Read the model definition and answer for the solid it produces. Units are mm, in the model's axes. Face numbers are marked on the shaded views. A direction names the side the tool comes from. Coordinates: 2 decimals unless noted, no trailing zeros. Loops run counter-clockwise (first coordinate to the right, second up) from the corner with the lowest first, then second, coordinate; pieces in that order, holes last. Notation, with made-up numbers: (-27, 11.5) -> (3, 11.5) arc R38 cw to (3, 49.5) -> close; hole circle Ø3 at (26, 59.5). An arc over 180 degrees is marked (long way). Answer in a Markdown table with one row per item.
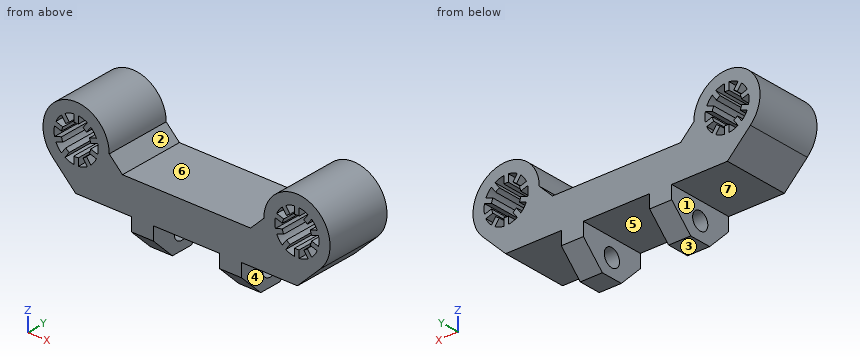
```python
from build123d import *

# Parameters (mm, degrees)
SKETCH1_R                      = 7.5
SKETCH1_R_2                    = 5
SKETCH1_W                      = 5
SKETCH1_H                      = 8
BOSS_EXTRUDE1_DEPTH            = 15
CHAMFER1_SIZE                  = 5
CUT_EXTRUDE1_REACH             = 42.293
SKETCH3_R                      = 2
CUT_EXTRUDE1_DIRECTION_2_REACH = 42.293


with BuildPart() as part:
    # Sketch1 → Boss-Extrude1 (new body)
    # profile 1 of 13: a face of its own
    with BuildSketch(Plane(origin=(0, 0, 0), x_dir=(1, 0, 0), z_dir=(0, 1, 0))):
        with Locations((-25, 0)):
            Circle(SKETCH1_R)
        with Locations((-25, 0)):
            Circle(SKETCH1_R_2, mode=Mode.SUBTRACT)
    # profile 2 of 13: a face of its own
    with BuildSketch(Plane(origin=(0, 0, 0), x_dir=(1, 0, 0), z_dir=(0, 1, 0))):
        with BuildLine():
            Line((-27.995843782, 1.499139764), (-29.576937931, 2.012868394))
            ThreePointArc((-29.576937931, 2.012868394), (-29.755282581, 1.545084972), (-29.885954926, 1.061811878))
            Line((-29.885954926, 1.061811878), (-28.304860777, 0.548083248))
            ThreePointArc((-28.304860777, 0.548083248), (-28.18603933, 1.035206931), (-27.995843782, 1.499139764))
        make_face()
    # profile 3 of 13: a face of its own
    with BuildSketch(Plane(origin=(0, 0, 0), x_dir=(1, 0, 0), z_dir=(0, 1, 0))):
        with BuildLine():
            Line((-28.304860777, -0.548083248), (-29.885954926, -1.061811878))
            ThreePointArc((-29.885954926, -1.061811878), (-29.755282581, -1.545084972), (-29.576937931, -2.012868394))
            Line((-29.576937931, -2.012868394), (-27.995843782, -1.499139764))
            ThreePointArc((-27.995843782, -1.499139764), (-28.18603933, -1.035206931), (-28.304860777, -0.548083248))
        make_face()
    # profile 4 of 13: a face of its own
    with BuildSketch(Plane(origin=(0, 0, 0), x_dir=(1, 0, 0), z_dir=(0, 1, 0))):
        with BuildLine():
            Line((-27.351533282, -2.385957087), (-28.328703206, -3.730916103))
            ThreePointArc((-28.328703206, -3.730916103), (-27.938926261, -4.045084972), (-27.519686212, -4.318701355))
            Line((-27.519686212, -4.318701355), (-26.542516288, -2.973742339))
            ThreePointArc((-26.542516288, -2.973742339), (-26.969080595, -2.710206931), (-27.351533282, -2.385957087))
        make_face()
    # profile 5 of 13: a face of its own
    with BuildSketch(Plane(origin=(0, 0, 0), x_dir=(1, 0, 0), z_dir=(0, 1, 0))):
        with BuildLine():
            Line((-25.5, -3.312476415), (-25.5, -4.974937186))
            ThreePointArc((-25.5, -4.974937186), (-25, -5), (-24.5, -4.974937186))
            Line((-24.5, -4.974937186), (-24.5, -3.312476415))
            ThreePointArc((-24.5, -3.312476415), (-25, -3.35), (-25.5, -3.312476415))
        make_face()
    # profile 6 of 13: a face of its own
    with BuildSketch(Plane(origin=(0, 0, 0), x_dir=(1, 0, 0), z_dir=(0, 1, 0))):
        with BuildLine():
            ThreePointArc((-22.480313788, -4.318701355), (-22.061073739, -4.045084972), (-21.671296794, -3.730916103))
            Line((-21.671296794, -3.730916103), (-22.648466718, -2.385957087))
            ThreePointArc((-22.648466718, -2.385957087), (-23.030919405, -2.710206931), (-23.457483712, -2.973742339))
            Line((-23.457483712, -2.973742339), (-22.480313788, -4.318701355))
        make_face()
    # profile 7 of 13: a face of its own
    with BuildSketch(Plane(origin=(0, 0, 0), x_dir=(1, 0, 0), z_dir=(0, 1, 0))):
        with BuildLine():
            ThreePointArc((-20.423062069, -2.012868394), (-20.244717419, -1.545084972), (-20.114045074, -1.061811878))
            Line((-20.114045074, -1.061811878), (-21.695139223, -0.548083248))
            ThreePointArc((-21.695139223, -0.548083248), (-21.81396067, -1.035206931), (-22.004156218, -1.499139764))
            Line((-22.004156218, -1.499139764), (-20.423062069, -2.012868394))
        make_face()
    # profile 8 of 13: a face of its own
    with BuildSketch(Plane(origin=(0, 0, 0), x_dir=(1, 0, 0), z_dir=(0, 1, 0))):
        with BuildLine():
            ThreePointArc((-20.114045074, 1.061811878), (-20.244717419, 1.545084972), (-20.423062069, 2.012868394))
            Line((-20.423062069, 2.012868394), (-22.004156218, 1.499139764))
            ThreePointArc((-22.004156218, 1.499139764), (-21.81396067, 1.035206931), (-21.695139223, 0.548083248))
            Line((-21.695139223, 0.548083248), (-20.114045074, 1.061811878))
        make_face()
    # profile 9 of 13: a face of its own
    with BuildSketch(Plane(origin=(0, 0, 0), x_dir=(1, 0, 0), z_dir=(0, 1, 0))):
        with BuildLine():
            ThreePointArc((-21.671296794, 3.730916103), (-22.061073739, 4.045084972), (-22.480313788, 4.318701355))
            Line((-22.480313788, 4.318701355), (-23.457483712, 2.973742339))
            ThreePointArc((-23.457483712, 2.973742339), (-23.030919405, 2.710206931), (-22.648466718, 2.385957087))
            Line((-22.648466718, 2.385957087), (-21.671296794, 3.730916103))
        make_face()
    # profile 10 of 13: a face of its own
    with BuildSketch(Plane(origin=(0, 0, 0), x_dir=(1, 0, 0), z_dir=(0, 1, 0))):
        with BuildLine():
            ThreePointArc((-24.5, 4.974937186), (-25, 5), (-25.5, 4.974937186))
            Line((-25.5, 4.974937186), (-25.5, 3.312476415))
            ThreePointArc((-25.5, 3.312476415), (-25, 3.35), (-24.5, 3.312476415))
            Line((-24.5, 3.312476415), (-24.5, 4.974937186))
        make_face()
    # profile 11 of 13: a face of its own
    with BuildSketch(Plane(origin=(0, 0, 0), x_dir=(1, 0, 0), z_dir=(0, 1, 0))):
        with BuildLine():
            Line((-26.542516288, 2.973742339), (-27.519686212, 4.318701355))
            ThreePointArc((-27.519686212, 4.318701355), (-27.938926261, 4.045084972), (-28.328703206, 3.730916103))
            Line((-28.328703206, 3.730916103), (-27.351533282, 2.385957087))
            ThreePointArc((-27.351533282, 2.385957087), (-26.969080595, 2.710206931), (-26.542516288, 2.973742339))
        make_face()
    # profile 12 of 13: a face of its own
    with BuildSketch(Plane(origin=(0, 0, 0), x_dir=(1, 0, 0), z_dir=(0, 1, 0))):
        with BuildLine():
            Line((-25.106601718, 10.5), (-30.303300859, 5.303300859))
            ThreePointArc((-30.303300859, 5.303300859), (-22.129874257, 6.929096494), (-17.5, 0))
            Line((-17.5, 0), (-14.5, 3))
            Line((-14.5, 3), (0, 3))
            Line((0, 3), (0, 10.5))
            Line((0, 10.5), (-7.5, 10.5))
            Line((-7.5, 10.5), (-12.5, 10.5))
            Line((-12.5, 10.5), (-25.106601718, 10.5))
        make_face()
    # profile 13 of 13: a face of its own
    with BuildSketch(Plane(origin=(0, 0, 0), x_dir=(1, 0, 0), z_dir=(0, 1, 0))):
        with Locations((-10, 14.5)):
            Rectangle(SKETCH1_W, SKETCH1_H)
    boss_extrude1 = extrude(amount=BOSS_EXTRUDE1_DEPTH)

    # Mirror1: Boss-Extrude1 across plane
    add(boss_extrude1.mirror(Plane(origin=(0, 0, 0), x_dir=(0, 0, 1), z_dir=(1, 0, 0))))

    # Chamfer1
    chamfer1_edges = [part.edges().sort_by_distance(p)[0] for p in [
        (10, 15, -18.5),
        (10, 0, -18.5),
        (-10, 15, -18.5),
        (-10, 0, -18.5),
    ]]
    chamfer(chamfer1_edges, length=CHAMFER1_SIZE)

    # Sketch3 → Cut-Extrude1 (cut, up to next)
    with BuildSketch(Plane(origin=(0, 0, 0), x_dir=(0, 0, -1), z_dir=(1, 0, 0)), mode=Mode.PRIVATE) as cut_extrude1_sk1:
        with Locations(Location((14.5, 7.5, 0), (0, 0, 180))):
            Circle(SKETCH3_R)
    cut_extrude1_tool1 = extrude(cut_extrude1_sk1.sketch, amount=-CUT_EXTRUDE1_REACH, mode=Mode.PRIVATE) & part.part
    add(cut_extrude1_tool1.solids().sort_by_distance((0, 7.5, -14.5))[0], mode=Mode.SUBTRACT)

    # Sketch3 → Cut-Extrude1 direction 2 (cut, up to next)
    with BuildSketch(Plane(origin=(0, 0, 0), x_dir=(0, 0, -1), z_dir=(1, 0, 0)), mode=Mode.PRIVATE) as cut_extrude1_direction_2_sk1:
        with Locations(Location((14.5, 7.5, 0), (0, 0, 180))):
            Circle(SKETCH3_R)
    cut_extrude1_direction_2_tool1 = extrude(cut_extrude1_direction_2_sk1.sketch, amount=CUT_EXTRUDE1_DIRECTION_2_REACH, mode=Mode.PRIVATE) & part.part
    add(cut_extrude1_direction_2_tool1.solids().sort_by_distance((0, 7.5, -14.5))[0], mode=Mode.SUBTRACT)


solid = part.part
```
1. A cutting plane is placed at D-D on x = 16.5. Give the vertices of the cut face in (y, z).
A:
| item | result |
|---|---|
| outline | (0, -10.5) -> (15, -10.5) -> (15, -1) -> (0, -1) -> close |
2. Find the intervals of material crossed by probe 1 along X at (y, z) = (13.25, -14.25); probe 2 along Z at (x, y) = (-8.9, 7.5); probe 3 along Z at (x, y) = (-18.5, 7.25), in increasing order.
A:
| item | result |
|---|---|
| probe 1 | x = -12.5 to -7.5, 7.5 to 12.5 |
| probe 2 | z = -18.5 to -16.5, -12.5 to -3 |
| probe 3 | z = -10.5 to 3.74 |
3. A cutting plane is placed at B-B on y = 7.5. Count the separate pieces of the cut face and the enclosed holes in it, and give its area (3 significant figures).
A:
| item | result |
|---|---|
| separate pieces | 3 |
| enclosed holes | 2 |
| area | 622 mm2 |
4. A cutting plane is placed at A-A on z = -14.5. Give the vertices of the cut face in (x, y).
A:
| item | result |
|---|---|
| outline | (-12.5, 1) -> (-7.5, 1) -> (-7.5, 5.5) -> (-12.5, 5.5) -> close; (-12.5, 9.5) -> (-7.5, 9.5) -> (-7.5, 14) -> (-12.5, 14) -> close; (7.5, 1) -> (12.5, 1) -> (12.5, 5.5) -> (7.5, 5.5) -> close; (7.5, 9.5) -> (12.5, 9.5) -> (12.5, 14) -> (7.5, 14) -> close |
5. A tool of negligible diameter and unlimited length cuts with its end or side. For the marked faces 4, 5, 6 and 7, from which of +Z, -Z, +X, -X, +Y, -Y can it reach the whole face along a straight path? Write none if from no direction.
A:
| item | result |
|---|---|
| face 4 | -Z, +X, +Y, -Y |
| face 5 | -Z, +Y, -Y |
| face 6 | +Z, +Y, -Y |
| face 7 | -Z, -X, +Y, -Y |
6. The mould has two halves that part along X. Classify the marked faces 1, 2 and 3: pulls with the +X half, pulls with the -X half, needs draft (parallel to the pull), parting line crosses it, or undercut.
A:
| item | result |
|---|---|
| face 1 | pulls with the -X half |
| face 2 | undercut |
| face 3 | needs draft |
7. Given pin 1 Ø0.8 at (y, z) = (5, -4) entering from +X; pin 2 Ø1.8 at (y, z) = (10, -4) entering from -X; pin 3 Ø2.5 at (y, z) = (10, -16) entering from +X; pin 4 Ø4 at (x, y) = (23, 8.5) entering from +Z, each flat-ended and moving along its own axis, determine where each tip first touches the part or whether it passes through.
A:
| item | result |
|---|---|
| pin 1 | stops at x = 31.58 |
| pin 2 | stops at x = -31.83 |
| pin 3 | stops at x = 12.5 |
| pin 4 | stops at z = 7.5 |
